Job drawing, mm, ordinate dimensions from the low corner. One solid piece. A direction names the side the tool comes from. Coordinates: 2 decimals unless noted, no trailing zeros. Write each loop counter-clockwise with the first axis right and the second up, starting at its lowest first coordinate (ties: lowest second). Pieces come first, ordered by that corner, then holes. Notation, with made-up numbers: (-28, 78.5) - (14, 78.5) arc R17 cw to (14, 95.5) - close; hole circle Ø7 at (-27.75, 7.5). An arc over 180 degrees is marked (long way). Put each result on its own line as item: value. Start each with the question number.
1. Saw through at B-B, the plane x = 50. Write the cut outline in (y, z), plus the area to 3 significant figures.
2. Saw through at C-C, the plane z = 25. Write the cut outline in (x, y).
3. Saw through at D-D, the plane y = 81. Write the cut outline in (x, z), plus the area to 3 significant figures.
4. Drop flat-ended pins along their axis: P1, Ø12, axis at x = 276.5, z = 93, coming from the -Y side; P2, Ø10, axis at y = 86.5, z = 132.5, coming from the +X side; P3, Ø2, axis at y = 87.5, z = 68, coming from the -X side. Give the stop position or say it passes through.
5. Drill centre lines: L1, parallel to Y at x = 514.5, z = 65; L2, parallel to Z at x = 50, y = 15; L3, parallel to X at y = 42, z = 16.5. Where is each one in solid material? Low to high. Write a range as from..to.
6. Which spindle directions (+Z, -Z, +X, -X, +Y, -Y) get a long thin tool onto all of the face, cutting with end or side? Do the marked faces 5, 6 and 7. Say none if no direction does.
7. Saw through at A-A, the plane z = 75. Write the cut outline in (x, y), plus the area to 3 significant figures.
8. Pull direction Y, two halves, no side cores. Call the marked faces 1, 2, 3 and 4: released by +Y, released by -Y, zero draft, split by the parting line, or undercut.
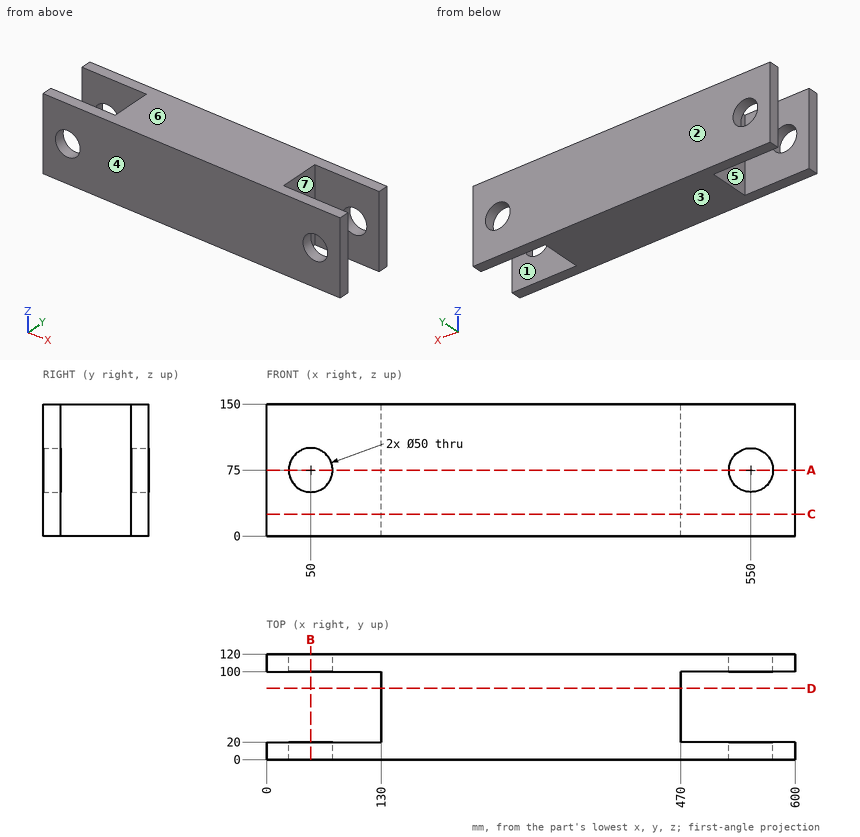
Final values:
1. outline: (0, 0) - (20, 0) - (20, 50) - (0, 50) - close; (0, 100) - (20, 100) - (20, 150) - (0, 150) - close; (100, 0) - (120, 0) - (120, 50) - (100, 50) - close; (100, 100) - (120, 100) - (120, 150) - (100, 150) - close
1. area: 4,000 mm²
2. outline: (0, 0) - (600, 0) - (600, 20) - (470, 20) - (470, 100) - (600, 100) - (600, 120) - (0, 120) - (0, 100) - (130, 100) - (130, 20) - (0, 20) - close
3. outline: (130, 0) - (470, 0) - (470, 150) - (130, 150) - close
3. area: 51,000 mm²
4. P1: stops at y = 0
4. P2: stops at x = 470
4. P3: stops at x = 130
5. L1: y = 0..20, 100..120
5. L2: z = 0..50, 100..150
5. L3: x = 130..470
6. face 5: +Z, -Z, -X
6. face 6: +Z, +X, -X, +Y, -Y
6. face 7: +Z, -Z, +X
7. outline: (0, 0) - (25, 0) - (25, 20) - (0, 20) - close; (0, 100) - (25, 100) - (25, 120) - (0, 120) - close; (75, 0) - (525, 0) - (525, 20) - (470, 20) - (470, 100) - (525, 100) - (525, 120) - (75, 120) - (75, 100) - (130, 100) - (130, 20) - (75, 20) - close; (575, 0) - (600, 0) - (600, 20) - (575, 20) - close; (575, 100) - (600, 100) - (600, 120) - (575, 120) - close
7. area: 47,200 mm²
8. face 1: undercut
8. face 2: released by +Y
8. face 3: zero draft
8. face 4: released by -Y
